Study the drawing (mm; zero at the part's minimum x, y, z) and answer. A direction names the side the tool comes from. Coordinates: 2 decimals unless noted, no trailing zeros. Loops run counter-clockwise (first coordinate to the right, second up) from the corner with the lowest first, then second, coordinate; pieces in that order, holes last. Notation, with made-up numbers: (86.5, -18) -> (98.5, -18) arc R29 cw to (98.5, 4) -> close; hole circle Ø2 at (-7, 69). An arc over 180 degrees is marked (long way). Answer as CSV lines item,"result".
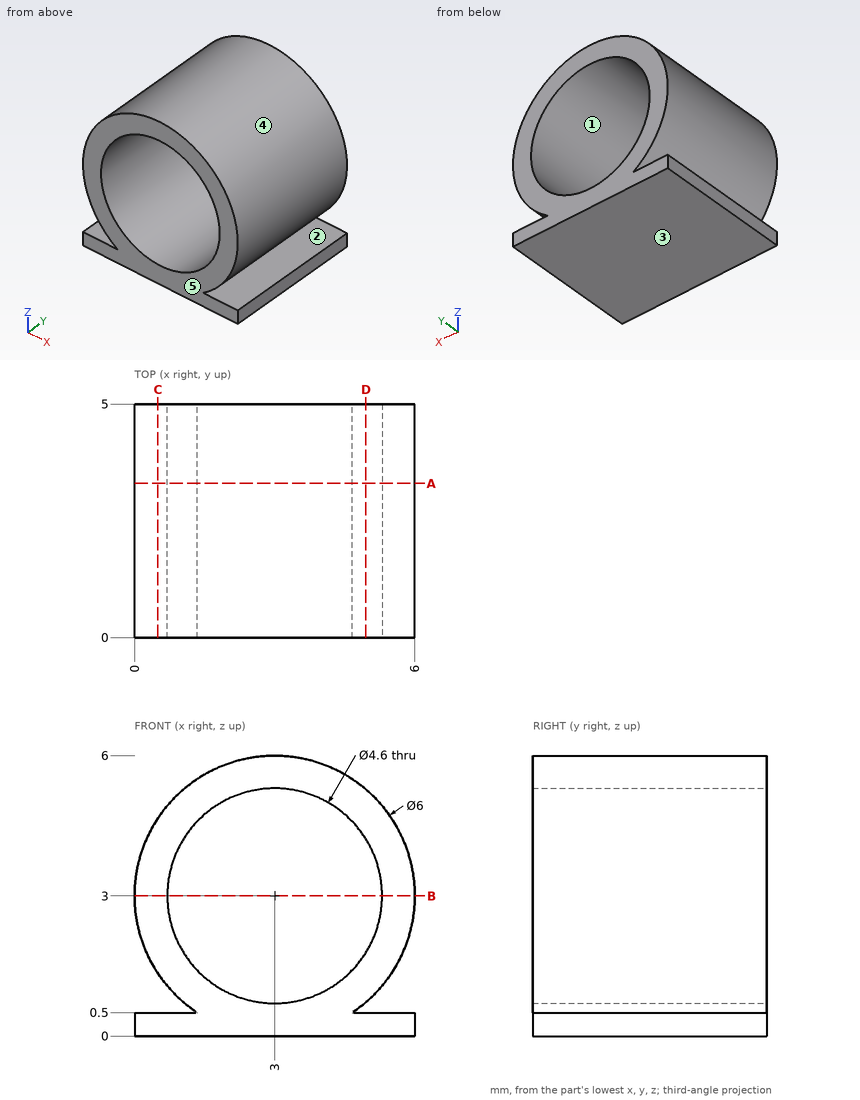
Q1. Given pin 1 Ø1.5 at (x, y) = (1, 3) entering from +Z; pin 2 Ø1.1 at (x, y) = (5.5, 2) entering from +Z, each flat-ended and moving along its own axis, determine where each tip first touches the part or whether it passes through.
Results:
pin 1,"stops at z = 5.73"
pin 2,"stops at z = 5.28"
Q2. For the marked faces 1 and 2, determine the directions among +Z, -Z, +X, -X, +Y, -Y from which every point of the face is accessible in a straight line to the end or side of a thin tool.
Results:
face 1,"+Y, -Y"
face 2,"+X, +Y, -Y"
Q3. For a pull along Z with two mould halves and no side action, classify the marked faces 3, 4 and 5 as pulls with the +Z half, pulls with the -Z half, needs draft (parallel to the pull), parting line crosses it, or undercut.
Results:
face 3,"pulls with the -Z half"
face 4,"undercut"
face 5,"needs draft"
Q4. A cutting plane is placed at B-B, the plane z = 3. Write down the section's boundary in (x, y), and give its area (3 significant figures).
Results:
outline,"(0, 0) -> (0.7, 0) -> (0.7, 5) -> (0, 5) -> close; (5.3, 0) -> (6, 0) -> (6, 5) -> (5.3, 5) -> close"
area,"7.00 mm²"
Q5. A cutting plane is placed at C-C, the plane x = 0.5. Write down the section's boundary in (y, z), and give its area (3 significant figures).
Results:
outline,"(0, 0) -> (5, 0) -> (5, 0.5) -> (0, 0.5) -> close; (0, 1.34) -> (5, 1.34) -> (5, 4.66) -> (0, 4.66) -> close"
area,"19.1 mm²"
Q6. Find the intervals of material crossed by probe 1 along Z at (x, y) = (3, 2.35); probe 2 along Z at (x, y) = (0.5, 3); probe 3 along X at (y, z) = (2.25, 3.5) (3 decimals), in increasing order. Write a range as [from, to].
Results:
probe 1,"z = [0, 0.7], [5.3, 6]"
probe 2,"z = [0, 0.5], [1.34, 4.66]"
probe 3,"x = [0.042, 0.755], [5.245, 5.958]"
Q7. A cutting plane is placed at D-D, the plane x = 4.95. Write down the section's boundary in (y, z), and give its area (3 significant figures).
Results:
outline,"(0, 0) -> (5, 0) -> (5, 0.5) -> (0, 0.5) -> close; (0, 0.72) -> (5, 0.72) -> (5, 1.78) -> (0, 1.78) -> close; (0, 4.22) -> (5, 4.22) -> (5, 5.28) -> (0, 5.28) -> close"
area,"13.1 mm²"
Q8. A cutting plane is placed at A-A, the plane y = 3.3. Write down the section's boundary in (x, z).
Results:
outline,"(0, 0) -> (6, 0) -> (6, 0.5) -> (4.66, 0.5) arc R3 ccw (long way) to (1.34, 0.5) -> (0, 0.5) -> close; hole circle Ø4.6 at (3, 3)"
